from build123d import *

# Parameters (mm, degrees)
F0_W     = 151.0536894202
F0_H     = 149.5463699102
F1_DEPTH = 60
F3_D     = 101.6
F2_R     = 50.8282360812
F4_DEPTH = 25.4
F8_R     = 5.08


# Not quite as in the source:
# - the program builds the solid bodies; features that only make, move or delete a surface that nothing else refers to are left out


with BuildPart() as f1:
    # F0 (on Top) → F1 (new body, symmetric)
    with BuildSketch(Plane.XY):
        with Locations((0.4253648221, 0.1466497779)):
            Rectangle(F0_W, F0_H)
    extrude(amount=F1_DEPTH, both=True)

    # F3 (through all)
    with Locations(Plane(origin=(0, 0, -60), x_dir=(1, 0, 0), z_dir=(0, 0, -1))):
        with Locations((0, 0)):
            Hole(F3_D / 2)

    # F2 (on face) → F4 (join)
    with BuildSketch(Plane(origin=(0, 0, -60), x_dir=(1, 0, 0), z_dir=(0, 0, -1))):
        Circle(F2_R)
    extrude(amount=-F4_DEPTH)

    # F8
    f8_edges = [f1.edges().sort_by_distance(p)[0] for p in [
        (-75.10148, 0.14665, 60),
        (0.425365, 74.919835, 60),
        (0.425365, -74.626535, 60),
        (75.95221, 0.14665, 60),
        (-50.8, 0, 60),
    ]]
    fillet(f8_edges, radius=F8_R)


solid = f1.part
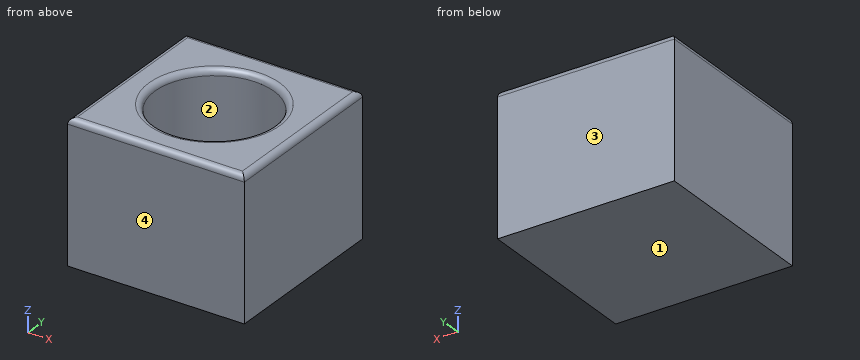
Design review of the part built by this model. Coordinates are the model's own, in mm. Face numbers are marked on the shaded views. Round coordinates to 2 decimals unless told otherwise and drop trailing zeros. Loops run counter-clockwise (first coordinate to the right, second up) from the corner with the lowest first, then second, coordinate; pieces in that order, holes last. Notation, with made-up numbers: (-10, -24.5) - (26, -24.5) arc R27 cw to (26, -3.5) - close; hole circle Ø5 at (-32, -37). An arc over 180 degrees is marked (long way). One line per item, written item: value. Start each with the question number.
1) To check wall thickness, follow L1, parallel to X at y = 0, z = 37; L2, parallel to Y at x = 2, z = 26; L3, parallel to Z at x = -6, y = -25. State the ranges of each line that lie inside material, in increasing order. Write a range as from..to.
2) Consider section C-C on z = 30. Give the boundary of the cut face in (x, y), then the cut area to 3 significant figures.
3) Draft analysis for pull direction Y (two halves, no side actions). For the marked faces 1, 2, 3 and 4, state which applies: +Y half, -Y half, draft (parallel to the pull), parting line (faces both ways), or undercut.
4) Consider section B-B on y = 0. Give the boundary of the cut face in (x, z), then the cut area to 3 significant figures.
5) Consider section A-A on x = 0. Give the boundary of the cut face in (y, z).
Reported:
1. L1: x = -75.1..-50.8, 50.8..75.95
1. L2: y = -74.63..-50.76, 50.76..74.92
1. L3: z = -60..-34.6
2. outline: (-75.1, -74.63) - (75.95, -74.63) - (75.95, 74.92) - (-75.1, 74.92) - close; hole circle Ø101.6 at (0, 0)
2. area: 14,500 mm^2
3. face 1: draft
3. face 2: undercut
3. face 3: +Y half
3. face 4: -Y half
4. outline: (-75.1, -60) - (75.95, -60) - (75.95, 54.92) arc R5.08 ccw to (70.87, 60) - (55.88, 60) arc R5.08 ccw to (50.8, 54.92) - (50.8, -34.6) - (-50.8, -34.6) - (-50.8, 54.92) arc R5.08 ccw to (-55.88, 60) - (-70.02, 60) arc R5.08 ccw to (-75.1, 54.92) - close
4. area: 8,490 mm^2
5. outline: (-74.63, -60) - (74.92, -60) - (74.92, 54.92) arc R5.08 ccw to (69.84, 60) - (55.88, 60) arc R5.08 ccw to (50.8, 54.92) - (50.8, -34.6) - (-50.8, -34.6) - (-50.8, 54.92) arc R5.08 ccw to (-55.88, 60) - (-69.55, 60) arc R5.08 ccw to (-74.63, 54.92) - close
